Geometry: final body of the model. Coordinates: model frame, mm. Face numbers are marked on the shaded views. A direction names the side the tool comes from. Round coordinates to 2 decimals unless told otherwise and drop trailing zeros. Loops run counter-clockwise (first coordinate to the right, second up) from the corner with the lowest first, then second, coordinate; pieces in that order, holes last. Notation, with made-up numbers: M 29,78.5 L 86,78.5 A26 ccw 86,112.5 Z; hole C -27.75,-20.75 d7. An arc over 180 degrees is marked long. Answer as a JSON object with one key per item and string values.
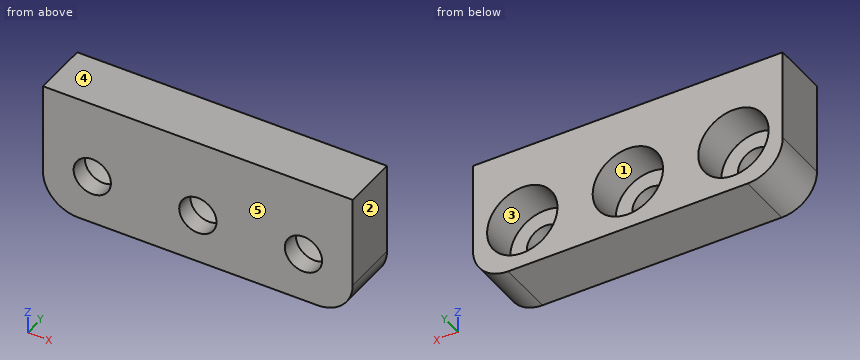
```python
from build123d import *

# Parameters (mm, degrees)
SKETCH1_W                                           = 44
SKETCH1_H                                           = 18
BOSS_EXTRUDE1_DEPTH                                 = 8
CBORE_FOR_M5_HEX_SOCKET_HEAD_CAP_SCREW1_D           = 5.3
CBORE_FOR_M5_HEX_SOCKET_HEAD_CAP_SCREW1_CBORE_D     = 10
CBORE_FOR_M5_HEX_SOCKET_HEAD_CAP_SCREW1_CBORE_DEPTH = 5.4
FILLET1_R                                           = 5


with BuildPart() as part:
    # Sketch1 → Boss-Extrude1 (new body)
    with BuildSketch(Plane(origin=(0, 0, 0), x_dir=(1, 0, 0), z_dir=(0, 1, 0))):
        Rectangle(SKETCH1_W, SKETCH1_H)
    extrude(amount=-BOSS_EXTRUDE1_DEPTH)

    # CBORE for M5 Hex Socket Head Cap Screw1 (through all)
    with Locations(Plane(origin=(0, 0, 0), x_dir=(1, 0, 0), z_dir=(0, 1, 0))):
        with Locations((-15, 2), (0, 2), (15, 2)):
            CounterBoreHole(CBORE_FOR_M5_HEX_SOCKET_HEAD_CAP_SCREW1_D / 2, CBORE_FOR_M5_HEX_SOCKET_HEAD_CAP_SCREW1_CBORE_D / 2, CBORE_FOR_M5_HEX_SOCKET_HEAD_CAP_SCREW1_CBORE_DEPTH)

    # Fillet1
    fillet1_edges = [part.edges().sort_by_distance(p)[0] for p in [
        (-22, -4, -9),
        (22, -4, -9),
    ]]
    fillet(fillet1_edges, radius=FILLET1_R)


solid = part.part
```
1) Line query: probe 1 along X at (y, z) = (-4.5, -2.25); probe 2 along Z at (x, y) = (0, -2.95); probe 3 along X at (y, z) = (-0.5, -0.25). Output: solid intervals per line, ascending.
Geometry results:
{"probe 1": "-22 to -19.99, -10.01 to -4.99, 4.99 to 10.01, 19.99 to 22", "probe 2": "-9 to -7, 3 to 9", "probe 3": "-22 to -19.68, -10.32 to -4.68, 4.68 to 10.32, 19.68 to 22"}
2) Cut plane D-D on z = 2. Return the cut outline in (x, y), and give its area (3 significant figures).
Geometry results:
{"outline": "M -22,-8 L 22,-8 L 22,0 L 18,0 L 18,-5.4 L 12,-5.4 L 12,0 L 3,0 L 3,-5.4 L -3,-5.4 L -3,0 L -12,0 L -12,-5.4 L -18,-5.4 L -18,0 L -22,0 Z", "area": "255 mm2"}
3) First-contact query: pin 1 (7 mm diameter, centred on x = 0, z = -2, fed in from +Y); pin 2 (5 mm diameter, centred on x = 15, z = -2, fed in from +Y). Flat tips, straight axial feed; report the tip coordinate or a pass-through.
Geometry results:
{"pin 1": "y = -5.4", "pin 2": "through"}
4) Cut plane C-C on x = -15. Return the cut outline in (y, z), and give its area (3 significant figures).
Geometry results:
{"outline": "M -8,-9 L 0,-9 L 0,-7 L -5.4,-7 L -5.4,-4.65 L -8,-4.65 Z; M -8,0.65 L -5.4,0.65 L -5.4,3 L 0,3 L 0,9 L -8,9 Z", "area": "76.2 mm2"}
5) Cut plane B-B on y = -7. Return the cut outline in (x, z).
Geometry results:
{"outline": "M -22,-4 A5 ccw -17,-9 L 17,-9 A5 ccw 22,-4 L 22,9 L -22,9 Z; hole C -15,-2 d5.3; hole C 0,-2 d5.3; hole C 15,-2 d5.3"}
6) Cut plane A-A on z = -2. Return the cut outline in (x, y), and give its area (3 significant figures).
Geometry results:
{"outline": "M -22,-8 L -17.65,-8 L -17.65,-5.4 L -20,-5.4 L -20,0 L -22,0 Z; M -12.35,-8 L -2.65,-8 L -2.65,-5.4 L -5,-5.4 L -5,0 L -10,0 L -10,-5.4 L -12.35,-5.4 Z; M 2.65,-8 L 12.35,-8 L 12.35,-5.4 L 10,-5.4 L 10,0 L 5,0 L 5,-5.4 L 2.65,-5.4 Z; M 17.65,-8 L 22,-8 L 22,0 L 20,0 L 20,-5.4 L 17.65,-5.4 Z", "area": "149 mm2"}
7) Pull-direction query (Z, two-part tool) for the marked faces 3, 4 and 5; classes: +Z half, -Z half, draft (parallel to the pull), parting line (faces both ways), or undercut.
Geometry results:
{"face 3": "undercut", "face 4": "+Z half", "face 5": "draft"}
8) Set-up query: the marked faces 1 and 2. Return all of +Z, -Z, +X, -X, +Y, -Y with unobstructed straight access to the full face (end or side cutting, diameter ignored); none if empty.
Geometry results:
{"face 1": "+Y", "face 2": "+Z, -Z, +X, +Y, -Y"}
